from build123d import *

# Parameters (mm, degrees)
SALIENTE_EXTRUIR1_DEPTH = 25
CROQUIS2_W              = 13.689149165
CROQUIS2_H              = 10.658244286
SALIENTE_EXTRUIR2_DEPTH = 8
REDONDEO1_R             = 0.5
CHAFL_N2_SIZE           = 2
CHAFL_N2_SIZE2          = 1.562571253
ESCALA2_SCALE           = 1.5
ESCALA3_SCALE           = 1.01
ESCALA4_SCALE           = 1.01
ESCALA5_SCALE           = 1.01


with BuildPart() as part:
    # Croquis1 → Saliente-Extruir1 (new body)
    with BuildSketch(Plane(origin=(0, 0, 0), x_dir=(0, 0, -1), z_dir=(1, 0, 0))):
        Polygon((6.829122143, 0), (-6.829122143, 0), (-6.829122143, 4), (0, 4.801857706), (6.829122143, 4), align=None)
    extrude(amount=SALIENTE_EXTRUIR1_DEPTH)

    # Croquis2 → Saliente-Extruir2 (add)
    with BuildSketch(Plane(origin=(0, 0, 0), x_dir=(1, 0, 0), z_dir=(0, 1, 0))):
        with Locations((6.844574583, 0)):
            Rectangle(CROQUIS2_W, CROQUIS2_H)
    extrude(amount=SALIENTE_EXTRUIR2_DEPTH)

    # Redondeo1
    redondeo1_edges = [part.edges().sort_by_distance(p)[0] for p in [
        (13.689149165, 4.488991896, 2.664561071),
        (13.689149165, 4.488991896, -2.664561071),
        (6.844574582, 4.176126087, 5.329122143),
        (6.844574582, 4.176126087, -5.329122143),
    ]]
    fillet(redondeo1_edges, radius=REDONDEO1_R)

    # Chaflán2
    chafl_n2_edges = [part.edges().sort_by_distance(p)[0] for p in [
        (0, 8, 0),
        (6.844574582, 8, 5.329122143),
        (13.689149165, 8, 0),
        (6.844574582, 8, -5.329122143),
    ]]
    chafl_n2_side = [part.faces().sort_by_distance(p)[0] for p in [
        (6.844574582, 8, 0),
    ]]
    chamfer(chafl_n2_edges, length=CHAFL_N2_SIZE, length2=CHAFL_N2_SIZE2, reference=chafl_n2_side[0])


with BuildPart() as part_1:
    # Escala2: scaled about (11.207296742, 3.085828341, 0)
    add(part.part.scale(ESCALA2_SCALE).moved(Location((-5.603648371, -1.542914171, 0))))


with BuildPart() as part_2:
    # Escala3: scaled about (11.207296743, 3.085828341, 0)
    add(part_1.part.scale(ESCALA3_SCALE).moved(Location((-0.112072967, -0.030858283, 0))))


with BuildPart() as part_3:
    # Escala4: scaled about (11.207296743, 3.085828341, 0)
    add(part_2.part.scale(ESCALA4_SCALE).moved(Location((-0.112072967, -0.030858283, 0))))


with BuildPart() as part_4:
    # Escala5: scaled about (11.207296743, 3.085828341, 0)
    add(part_3.part.scale(ESCALA5_SCALE).moved(Location((-0.112072967, -0.030858283, 0))))


solid = part_4.part
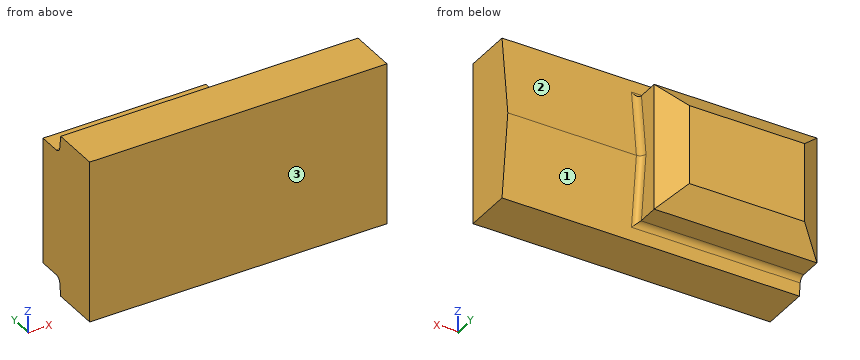
Design review of the part built by this model. Coordinates are the model's own, in mm. Face numbers are marked on the shaded views. A direction names the side the tool comes from. Give positions to 0.01 mm unless a question says otherwise; leave off trailing zeros. Order: outer loops, then holes, each group sorted by start corner. A loop starts at its lowest first (then second) coordinate and runs counter-clockwise, first axis right, second up. Notation, with made-up numbers: (23, 41.5) - (77, 41.5) arc R15 ccw to (77, 47.5) - close; hole circle Ø11 at (-8, 45). An arc over 180 degrees is marked (long way). Write item = value, one per line. Start each with the question number.
Q1. We need section A-A on x = -1.5. State the section outline as (y, z) points (3 decimals), plus the area to 3 significant figures.
Q2. Tool access review of the marked faces 1, 2 and 3: name each direction out of +Z, -Z, +X, -X, +Y, -Y from which nothing blocks a thin tool from reaching the whole face with its end or side.
Q3. We need section B-B on x = 28.5. State the section outline as (y, z) points, plus the area to 3 significant figures.
Q4. To check wall thickness, follow L1, parallel to X at y = 7.25, z = -0.75; L2, parallel to Y at x = 8, z = -6; L3, parallel to X at y = 9, z = -4.5. State the ranges of each line that lie inside material, in increasing order. Write a range as from..to.
Q5. Clearance check with flat-ended pins moving along their axes: pin 1 Ø2 at (x, y) = (0, 7.5) entering from +Z; pin 2 Ø1.4 at (x, y) = (7.5, 6.5) entering from -Z. State where each tip first meets the part, or that it passes through.
Working result:
q1.outline = (-1.683, -10.554) - (4.499, -10.554) - (4.691, -8.919) arc R0.773 cw to (5.458, -8.236) - (8.266, -8.236) - (10.68, -5.145) - (10.68, 5.145) - (8.266, 8.236) - (5.458, 8.236) arc R0.773 cw to (4.691, 8.919) - (4.499, 10.554) - (-1.683, 10.554) - close
q1.area = 226 mm²
q2.face_1 = -Z, +X, +Y
q2.face_2 = +Z, +X, +Y
q2.face_3 = +Z, -Z, +X, -X, -Y
q3.outline = (-1.68, -10.55) - (4.5, -10.55) - (5.74, 0) - (4.5, 10.55) - (-1.68, 10.55) - close
q3.area = 144 mm²
q4.L1 = -6.11..15.04
q4.L2 = -1.68..10.01
q4.L3 = -5.17..14.1
q5.pin_1 = 8.24
q5.pin_2 = -8.24
